from build123d import *

# Parameters (mm, degrees)
SKETCH1_R           = 19
SKETCH1_R_2         = 2.6
BOSS_EXTRUDE1_DEPTH = 5
SKETCH2_R           = 4.4
CUT_EXTRUDE1_DEPTH  = 3
BOSS_EXTRUDE2_DEPTH = 25
FILLET1_R           = 0.5
SKETCH4_R           = 2.05
CUT_EXTRUDE2_DEPTH  = 45.184100423


with BuildPart() as part:
    # Sketch1 → Boss-Extrude1 (new body)
    with BuildSketch(Plane(origin=(0, 0, 0), x_dir=(1, 0, 0), z_dir=(0, 1, 0))):
        with Locations(Location((0, 0, 0), (0, 0, 270))):
            Circle(SKETCH1_R)
        with Locations(Location((11.691342951, 6.75, 0), (0, 0, 270))):
            Circle(SKETCH1_R_2, mode=Mode.SUBTRACT)
        with Locations(Location((11.691342951, -6.75, 0), (0, 0, 270))):
            Circle(SKETCH1_R_2, mode=Mode.SUBTRACT)
        with Locations(Location((-11.691342951, -6.75, 0), (0, 0, 270))):
            Circle(SKETCH1_R_2, mode=Mode.SUBTRACT)
        with Locations(Location((-11.691342951, 6.75, 0), (0, 0, 270))):
            Circle(SKETCH1_R_2, mode=Mode.SUBTRACT)
    extrude(amount=BOSS_EXTRUDE1_DEPTH)

    # Sketch2 → Cut-Extrude1 (cut)
    with BuildSketch(Plane(origin=(0, 5, 0), x_dir=(1, 0, 0), z_dir=(0, 1, 0))):
        with Locations(Location((-11.691342951, 6.75, 0), (0, 0, 270))):
            Circle(SKETCH2_R)
        with Locations(Location((11.691342951, 6.75, 0), (0, 0, 270))):
            Circle(SKETCH2_R)
        with Locations(Location((11.691342951, -6.75, 0), (0, 0, 270))):
            Circle(SKETCH2_R)
        with Locations(Location((-11.691342951, -6.75, 0), (0, 0, 270))):
            Circle(SKETCH2_R)
    extrude(amount=-CUT_EXTRUDE1_DEPTH, mode=Mode.SUBTRACT)

    # Sketch3 → Boss-Extrude2 (add)
    with BuildSketch(Plane(origin=(0, 5, 0), x_dir=(1, 0, 0), z_dir=(0, 1, 0))):
        with BuildLine():
            Line((-7.291342951, 17.54526483), (-7.291342951, -17.54526483))
            ThreePointArc((-7.291342951, -17.54526483), (0, -19), (7.291342951, -17.54526483))
            Line((7.291342951, -17.54526483), (7.291342951, 17.54526483))
            ThreePointArc((7.291342951, 17.54526483), (0, 19), (-7.291342951, 17.54526483))
        make_face()
    extrude(amount=BOSS_EXTRUDE2_DEPTH)

    # Fillet1
    fillet1_edges = [part.edges().sort_by_distance(p)[0] for p in [
        (0, 30, -19),
        (-7.291342951, 30, 0),
        (0, 30, 19),
        (7.291342951, 30, 0),
    ]]
    fillet(fillet1_edges, radius=FILLET1_R)

    # Sketch4 → Cut-Extrude2 (cut, through all)
    with BuildSketch(Plane(origin=(7.291342951, 0, 0), x_dir=(0, 0, -1), z_dir=(1, 0, 0))):
        with Locations((-12.54526483, 23.375)):
            Circle(SKETCH4_R)
        with Locations((12.54526483, 23.375)):
            Circle(SKETCH4_R)
        with Locations((0, 17.25)):
            Circle(SKETCH4_R)
    extrude(amount=-CUT_EXTRUDE2_DEPTH, mode=Mode.SUBTRACT)


solid = part.part
Geometry: final body of the model. Coordinates: model frame, mm. A direction names the side the tool comes from. Give positions to 0.01 mm unless a question says otherwise; leave off trailing zeros. Write each loop counter-clockwise with the first axis right and the second up, starting at its lowest first coordinate (ties: lowest second). Pieces come first, ordered by that corner, then holes. Notation, with made-up numbers: M 14.25,-27 L 34.25,-27 A5 ccw 34.25,-20 Z; hole C -38.5,-5 d2. An arc over 180 degrees is marked long. Answer in a Markdown table with one row per item. Add a question column.
(1) Section C-C on y = 22. Return loops of the section in (x, z).
(2) Ray query, line 1 (Z direction, x = -13, y = 4.5); line 2 (X direction, y = 1.5, z = 6.75); line 3 (X direction, y = 3.2, z = 6.75). Return the intervals inside material, ascending.
(3) First-contact query: pin 1 (5.5 mm diameter, centred on y = 17.25, z = 0, fed in from +X); pin 2 (8 mm diameter, centred on x = -11.69, z = -6.75, fed in from +Y); pin 3 (7 mm diameter, centred on x = 13.5, z = -7.5, fed in from +Y); pin 4 (7 mm diameter, centred on x = 11.69, z = 6.75, fed in from -Y). Flat tips, straight axial feed; report the tip coordinate or a pass-through.
(4) Section D-D on z = -5. Return loops of the section in (x, y), and give its area (3 significant figures).
(5) Mould query, pull axis Y, two halves, no side actions, for faces 1 (the cylindrical face through (-10.91, 0.99, -4.27)), 2 (the flat face through (-14, 2, 9)), 3 (the cylindrical face through (0.102, 18.635, 1.511)). Classes: +Y half, -Y half, draft (parallel to the pull), parting line (faces both ways), or undercut.
(6) Reachability of faces 4 (the cylindrical face through (0.1, 23.99, -14.5)), 5 (the flat face through (-12, 5, 0)), 6 (the cylindrical face through (-9.113, 0.986, 6.412)), 7 (the flat face through (13, 5, 0)), 8 (the cylindrical face through (15.4, 3.52, 9.12)) from +Z, -Z, +X, -X, +Y, -Y: full face, straight path, thin tool, end or side. Return the list, or none.
(7) Section A-A on y = 17.25. Return loops of the section in (x, z).
(8) Section B-B on z = 13. Return loops of the section in (x, y), and give its area (3 significant figures).
Result set:
| question | item | result |
|---|---|---|
| 1 | outline | M -7.29,-17.55 A19 ccw 7.29,-17.55 L 7.29,-14.07 L -7.29,-14.07 Z; M -7.29,-11.02 L 7.29,-11.02 L 7.29,11.02 L -7.29,11.02 Z; M -7.29,14.07 L 7.29,14.07 L 7.29,17.55 A19 ccw -7.29,17.55 Z |
| 2 | line 1 | z = -13.86 to -10.95, -2.55 to 2.55, 10.95 to 13.86 |
| 2 | line 2 | x = -17.76 to -14.29, -9.09 to 9.09, 14.29 to 17.76 |
| 2 | line 3 | x = -17.76 to -16.09, -7.29 to 7.29, 16.09 to 17.76 |
| 3 | pin 1 | stops at x = 7.29 |
| 3 | pin 2 | stops at y = 2 |
| 3 | pin 3 | stops at y = 5 |
| 3 | pin 4 | stops at y = 0 |
| 4 | outline | M -18.33,0 L -13.61,0 L -13.61,2 L -15.73,2 L -15.73,5 L -18.33,5 Z; M -9.77,0 L 9.77,0 L 9.77,2 L 7.65,2 L 7.65,5 L 7.29,5 L 7.29,29.5 A0.5 ccw 6.79,30 L -6.79,30 A0.5 ccw -7.29,29.5 L -7.29,5 L -7.65,5 L -7.65,2 L -9.77,2 Z; M 13.61,0 L 18.33,0 L 18.33,5 L 15.73,5 L 15.73,2 L 13.61,2 Z |
| 4 | area | 484 mm^2 |
| 5 | face 1 | draft |
| 5 | face 2 | +Y half |
| 5 | face 3 | undercut |
| 6 | face 4 | +X, -X |
| 6 | face 5 | +Z, -Z, -X, +Y |
| 6 | face 6 | +Y, -Y |
| 6 | face 7 | +Z, -Z, +X, +Y |
| 6 | face 8 | +Y |
| 7 | outline | M -7.29,-17.55 A19 ccw 7.29,-17.55 L 7.29,-2.05 L -7.29,-2.05 Z; M -7.29,2.05 L 7.29,2.05 L 7.29,17.55 A19 ccw -7.29,17.55 Z |
| 8 | outline | M -13.86,0 L 13.86,0 L 13.86,5 L 7.29,5 L 7.29,21.38 L -7.29,21.38 L -7.29,5 L -13.86,5 Z; M -7.29,25.37 L 7.29,25.37 L 7.29,29.5 A0.5 ccw 6.79,30 L -6.79,30 A0.5 ccw -7.29,29.5 Z |
| 8 | area | 445 mm^2 |
